Check sheet for the modelled part. Datum: model origin and axes. Units: mm. Coordinates: 2 decimals unless noted, no trailing zeros. Loops run counter-clockwise (first coordinate to the right, second up) from the corner with the lowest first, then second, coordinate; pieces in that order, holes last. Notation, with made-up numbers: (64.5, 63.5) -> (95.5, 63.5) arc R22 cw to (95.5, 87.5) -> close; hole circle Ø6 at (52.25, -27). An arc over 180 degrees is marked (long way). Use CSV: the item, a comma, the result in double quotes.
Autodesk Inventor part; units mm, degrees
ref_plane "YZ Plane" through (0, 0, 0) normal (1, 0, 0) x (0, 1, 0)
ref_plane "XZ Plane" through (0, 0, 0) normal (0, 1, 0) x (-1, 0, 0)
ref_plane "XY Plane" through (0, 0, 0) normal (0, 0, 1) x (1, 0, 0)
sketch "Sketch1" plane through (0, 0, 0) normal (1, 0, 0) x (0, 1, 0)
  circle A0 centre (0, 0) radius 7.5075
  circle A1 centre (-56.0605, -56.0605) radius 2.65
  circle A2 centre (-38.1, -38.1) radius 2.65
  circle A3 centre (-47.0803, 100.9618) radius 2.65
  circle A4 centre (-56.0605, 109.942) radius 2.65
  circle A5 centre (-38.1, 91.9815) radius 2.65
  circle A6 centre (-47.0803, -47.0803) radius 2.65
  line L0 (-47.0803, 100.9618) -> (6.8013, 47.0803) construction
  line L1 (-35.921, 35.921) -> (0, 0) construction
  line L2 (0, 0) -> (-35.921, -35.921) construction
  line L3 (0, 0) -> (12.7, 0) construction
  line L4 (-47.0803, 118.9223) -> (15.3303, 56.5118)
  line L5 (19.05, 47.5315) -> (19.05, 6.35)
  line L6 (-68.7605, -56.0605) -> (-68.7605, 109.942)
  arc A7 (19.05, 47.5315) -> (15.3303, 56.5118) centre (6.35, 47.5315) ccw
  arc A8 (-47.0803, 118.9223) -> (-68.7605, 109.942) centre (-56.0605, 109.942) ccw
  line L7 (-47.0803, -65.0408) -> (15.3303, -2.6303)
  arc A9 (15.3303, -2.6303) -> (19.05, 6.35) centre (6.35, 6.35) ccw
  arc A10 (-68.7605, -56.0605) -> (-47.0803, -65.0408) centre (-56.0605, -56.0605) ccw
  line L8 (-26.9408, -8.9802) -> (-44.9013, -26.9407)
  line L9 (-44.9013, -26.9407) -> (-284.0015, 212.1595)
  line L10 (-266.041, 230.12) -> (-284.0015, 212.1595)
  line L11 (-26.9408, -8.9802) -> (-266.041, 230.12)
  circle A11 centre (-56.0605, 2.179) radius 2.65
  circle A12 centre (-44.9013, -8.9802) radius 2.65
  line L12 (-56.0605, 2.179) -> (-44.9013, -8.9802) construction
  point P0 (19.05, 1.0895)
  point P1 (-68.7605, -86.721)
  point P2 (-68.7605, 32.8395)
  dimension "d0" = 15.015
  dimension "d1" = 5.3
  dimension "d2" = 5.3
  dimension "d3" = 5.3
  dimension "d4" = 5.3
  dimension "d5" = 5.3
  dimension "d6" = 5.3
  dimension "d8" = 38.1
  dimension "d10" = 38.1
  dimension "d11" = 12.7
  dimension "d12" = 12.7
  dimension "d13" = 38.1
  dimension "d14" = 12.7
  dimension "d15" = 12.7
  dimension "d16" = 12.7
  dimension "d18" = 19.05
  dimension "d19" = 45
  dimension "d20" = 12.7
  dimension "d21" = 12.7
  dimension "d24" = 12.7
  dimension "d25" = 12.7
  dimension "d27" = 12.7
  dimension "d29" = 12.7
  dimension "d34" = 12.7
  dimension "d47" = 12.7
  dimension "d49" = 50.8
  dimension "d50" = 76.2
  dimension "d51" = 12.7
extrude "Extrusion2" add sketch "Sketch1" along normal blind 3.175 contours A3 | A6 | L4 A7 L5 A9 L7 A10 L6 L9 L8 L11 A8 | L11 L8 L9 L6
sketch "Sketch3" plane through (3.175, 0, 0) normal (1, 0, 0) x (0, 0, -1)
  circle A0 centre (0, 0) radius 7.5075
  circle A1 centre (0, 0) radius 13 construction
  circle A2 centre (-0.0008, 13) radius 2
  line L0 (-6.35, 19.05) -> (-47.5315, 19.05)
  circle A3 centre (-13, -0.0008) radius 2
  circle A4 centre (0.0008, -13) radius 2
  circle A5 centre (13, 0.0008) radius 2
  dimension "d37" = 26
  dimension "d38" = 4
  dimension "d42" = 360
extrude "Extrusion3" cut sketch "Sketch3" against normal blind 25.4 contours A2 | A3 | A4 | A5
equation "\"d12\" = d11"
equation "\"d14\" = d11"
equation "\"d15\" = d11"
properties part number "HipPivotPlate" material "Aluminum 6061"
1) Thickness scan on line 1 along Y through (x, z) = (2.4, 13); line 2 along Y through (x, z) = (2.7, 3); line 3 along Z through (x, y) = (2.3, -12). Record the ranges inside material, lowest first. Write a range as from..to.
Answer below:
line 1,"y = -68.76..-2, 2..19.05"
line 2,"y = -68.76..-58.58, -53.54..-6.88, 6.88..18.6"
line 3,"z = -29.96..-1.73, 1.73..83.84"
2) Cross-section at B-B on y = -13. Record the boundary of the cut face in (x, z) (3 decimals).
Answer below:
outline,"(0, -30.961) -> (3.175, -30.961) -> (3.175, -2.001) -> (0, -2.001) -> close; (0, 1.999) -> (3.175, 1.999) -> (3.175, 84.842) -> (0, 84.842) -> close"
3) Cross-section at D-D on x = 1.2. Give the number of separate pieces and of enclosed holes in the cut face, and give its area (3 significant figures).
Answer below:
separate pieces,"1"
enclosed holes,"11"
area,"11,500 mm²"
4) Cross-section at C-C on y = -57. Record the boundary of the cut face in (x, z) (3 decimals), and give its area (3 significant figures).
Answer below:
outline,"(0, -68.726) -> (3.175, -68.726) -> (3.175, -58.538) -> (0, -58.538) -> close; (0, -53.583) -> (3.175, -53.583) -> (3.175, -0.299) -> (0, -0.299) -> close; (0, 4.657) -> (3.175, 4.657) -> (3.175, 107.464) -> (0, 107.464) -> close; (0, 112.42) -> (3.175, 112.42) -> (3.175, 122.607) -> (0, 122.607) -> close"
area,"560 mm²"
5) Draft check along Y on faces 1 (the flat face through (2, -68.76, 26)), 2 (the cylindrical face through (1.565, -58.708, -56.177)), 3 (the flat face through (0, -35, 28)). Enter one of: released by +Y, released by -Y, zero draft, split by the parting line, or undercut.
Answer below:
face 1,"released by -Y"
face 2,"undercut"
face 3,"zero draft"
